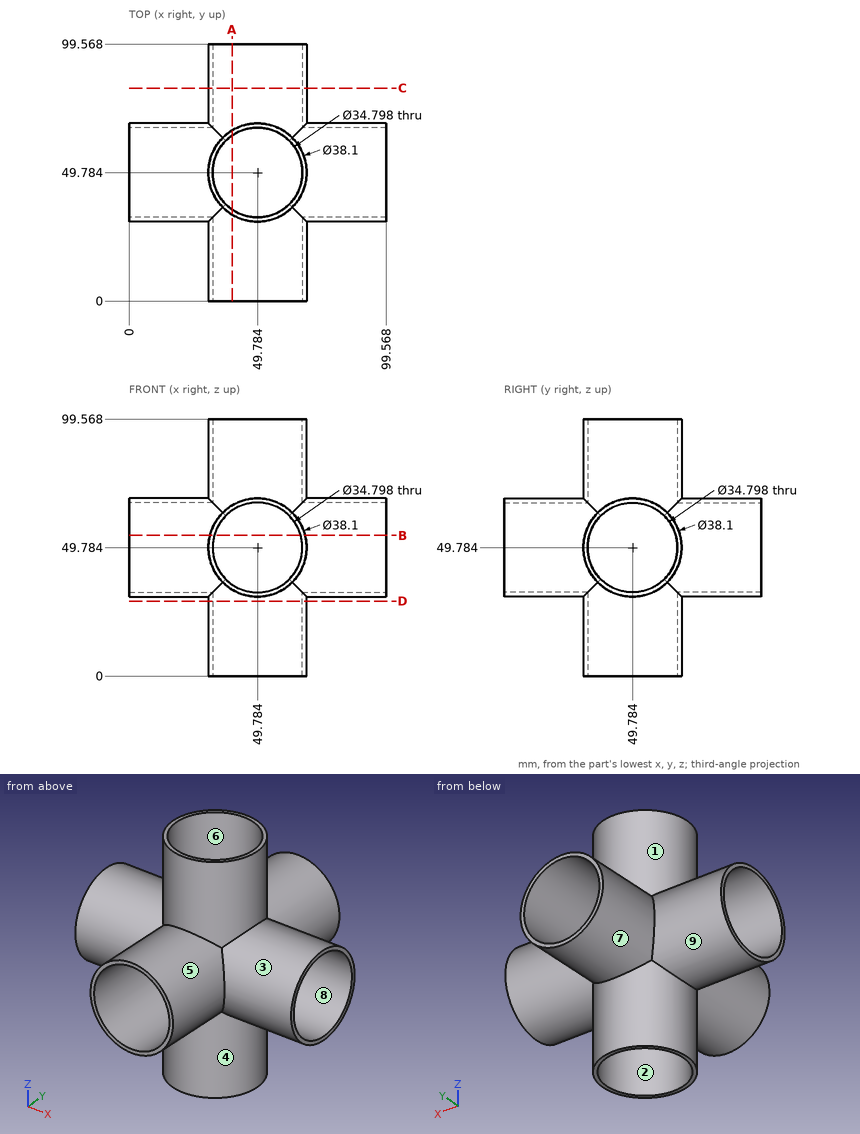
Here's the drawing with two shaded views (mm, measured from the low corner). I have some questions. A direction names the side the tool comes from. Coordinates: 2 decimals unless noted, no trailing zeros. Loops run counter-clockwise (first coordinate to the right, second up) from the corner with the lowest first, then second, coordinate; pieces in that order, holes last. Notation, with made-up numbers: (35.5, 67) - (88.5, 67) arc R31 ccw to (88.5, 92) - close; hole circle Ø6 at (-38, -3). An arc over 180 degrees is marked (long way). Answer as CSV lines item,"result". Start each with the question number.
1) Suppose I cut it at C-C (y = 82.5). Please give me the cut outline in (x, z), plus the area to 3 significant figures.
2) Suppose I cut it at B-B (z = 54.5). Please give me the cut outline in (x, y).
3) I need wall thicknesses on line 1 (Y direction, x = 25.5, z = 49); line 2 (X direction, y = 19, z = 49.5); line 3 (Z direction, x = 77.5, y = 62). Which ranges of each line are inside material? Lowest first, please. Write a range as from..to.
4) Which directions (+Z, -Z, +X, -X, +Y, -Y) give clear straight access to the entire face, cutting with the end or side of a thin tool? Please do the marked faces 1, 2, 3, 4 and 5.
5) Thinking about a two-plate mould opening in Y: for the marked faces 6, 7, 8 and 9, which applies, pulls with the +Y half, pulls with the -Y half, needs draft (parallel to the pull), parting line crosses it, or undercut?
6) Suppose I cut it at A-A (x = 40). Please give me the cut outline in (y, z), plus the area to 3 significant figures.
7) For pin 1 (1.5 mm diameter, centred on x = 60, y = 17, fed in from -Z); pin 2 (21 mm diameter, centred on y = 49.784, z = 49.784, fed in from -X); pin 3 (2 mm diameter, centred on x = 32.5, y = 24, fed in from -Z); pin 4 (10 mm diameter, centred on y = 72, z = 66.5, fed in from +X), each with a flat end and sliding along its axis, tell me the tip position at first contact or that it passes through.
Check result:
1,outline,"circle Ø38.1 at (49.78, 49.78); hole circle Ø34.8 at (49.78, 49.78)"
1,area,"189 mm²"
2,outline,"(0, 31.33) - (31.33, 31.33) - (31.33, 0) - (33.04, 0) - (33.04, 33.04) - (0, 33.04) - close; (0, 66.53) - (33.04, 66.53) - (33.04, 99.57) - (31.33, 99.57) - (31.33, 68.24) - (0, 68.24) - close; (66.53, 0) - (68.24, 0) - (68.24, 31.33) - (99.57, 31.33) - (99.57, 33.04) - (66.53, 33.04) - close; (66.53, 66.53) - (99.57, 66.53) - (99.57, 68.24) - (68.24, 68.24) - (68.24, 99.57) - (66.53, 99.57) - close"
3,line 1,"y = 30.75..32.4, 67.17..68.82"
3,line 2,"x = 30.74..32.39, 67.18..68.83"
3,line 3,"z = 35.17..37.39, 62.17..64.4"
4,face 1,"+Z"
4,face 2,"+Z, -Z"
4,face 3,"+X"
4,face 4,"-Z"
4,face 5,"-Y"
5,face 6,"undercut"
5,face 7,"needs draft"
5,face 8,"undercut"
5,face 9,"parting line crosses it"
6,outline,"(0, 33.44) - (33.44, 33.44) - (33.44, 0) - (35.4, 0) - (35.4, 35.4) - (0, 35.4) - close; (0, 64.17) - (35.4, 64.17) - (35.4, 99.57) - (33.44, 99.57) - (33.44, 66.13) - (0, 66.13) - close; (64.17, 0) - (66.13, 0) - (66.13, 33.44) - (99.57, 33.44) - (99.57, 35.4) - (64.17, 35.4) - close; (64.17, 64.17) - (99.57, 64.17) - (99.57, 66.13) - (66.13, 66.13) - (66.13, 99.57) - (64.17, 99.57) - close"
6,area,"539 mm²"
7,pin 1,"stops at z = 33.25"
7,pin 2,"passes through"
7,pin 3,"stops at z = 39.9"
7,pin 4,"stops at x = 64.81"
